Drawing for the job (mm, zero at the part's lowest x, y, z). A direction names the side the tool comes from. Coordinates: 2 decimals unless noted, no trailing zeros. Write each loop counter-clockwise with the first axis right and the second up, starting at its lowest first coordinate (ties: lowest second). Pieces come first, ordered by that corner, then holes. Notation, with made-up numbers: (-10.5, 2.5) -> (-1.5, 2.5) arc R9 ccw to (-1.5, 13.5) -> close; hole circle Ø8 at (80.5, 80.25). An arc over 180 degrees is marked (long way). Write each question's results on one line, items separated by ' | '. Start each with the question number.
Q1. Saw through at D-D on x = 46.5. Give the cut face in (y, z).
Q2. Saw through at C-C on z = 11. Give the cut face in (x, y).
Q3. Saw through at B-B on x = 31. Give the cut face in (y, z), and give its area (3 significant figures).
Q4. Drop a flat-ended pin along its axis: pin 1 Ø15 at (x, z) = (25, 14) entering from +Y. Give the stop position or say it passes through.
Q5. Drill centre lines: line 1 (X direction, y = 6.25, z = 25); line 2 (X direction, y = 13, z = 26); line 3 (Y direction, x = 42, z = 21.5). Where is each one in solid material? Low to high.
Q6. Two-plate mould, pull along X, no slides. Class the marked faces 1, 2 and 3: released by +X, released by -X, zero draft, split by the parting line, or undercut.
Q7. Saw through at A-A on y = 28. Give the cut face in (x, z).
Q8. Tool access for the marked faces 4, 5 and 6: list every direction of +Z, -Z, +X, -X, +Y, -Y with a clear straight run to the whole face (end or side of a thin tool).
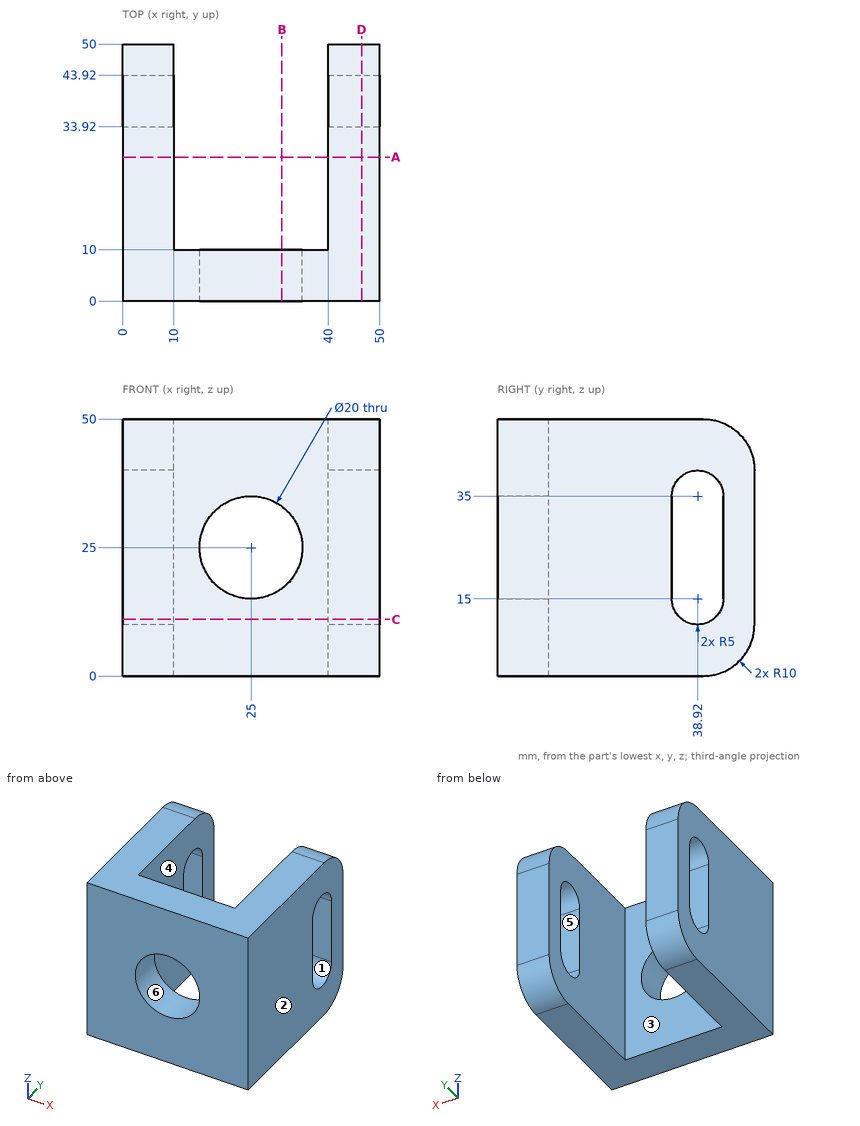
Returned:
1) outline: (0, 0) -> (40, 0) arc R10 ccw to (50, 10) -> (50, 40) arc R10 ccw to (40, 50) -> (0, 50) -> close; hole (33.92, 15) arc R5 ccw to (43.92, 15) -> (43.92, 35) arc R5 ccw to (33.92, 35) -> close
2) outline: (0, 0) -> (50, 0) -> (50, 35.92) -> (40, 35.92) -> (40, 10) -> (10, 10) -> (10, 35.92) -> (0, 35.92) -> close; (0, 41.92) -> (10, 41.92) -> (10, 50) -> (0, 50) -> close; (40, 41.92) -> (50, 41.92) -> (50, 50) -> (40, 50) -> close
3) outline: (0, 0) -> (10, 0) -> (10, 17) -> (0, 17) -> close; (0, 33) -> (10, 33) -> (10, 50) -> (0, 50) -> close | area: 340 mm2
4) pin 1: stops at y = 10
5) line 1: x = 0 to 15, 35 to 50 | line 2: x = 0 to 10, 40 to 50 | line 3: y = 0 to 33.92, 43.92 to 50
6) face 1: zero draft | face 2: released by +X | face 3: undercut
7) outline: (0, 0) -> (10, 0) -> (10, 50) -> (0, 50) -> close; (40, 0) -> (50, 0) -> (50, 50) -> (40, 50) -> close
8) face 4: +Z, -Z, +Y | face 5: +X, -X | face 6: +Y, -Y
